Answer from the drawing. Dimensions are ordinates in mm from the lowest x, y and z of the part. Round coordinates to 2 decimals unless told otherwise and drop trailing zeros. Loops run counter-clockwise (first coordinate to the right, second up) from the corner with the lowest first, then second, coordinate; pieces in that order, holes last. Notation, with made-up numbers: M 8,7.5 L 42,7.5 A6 ccw 42,14.5 Z; hole C -5.5,39.25 d4. An arc over 180 degrees is marked long. One line per item, written item: value.
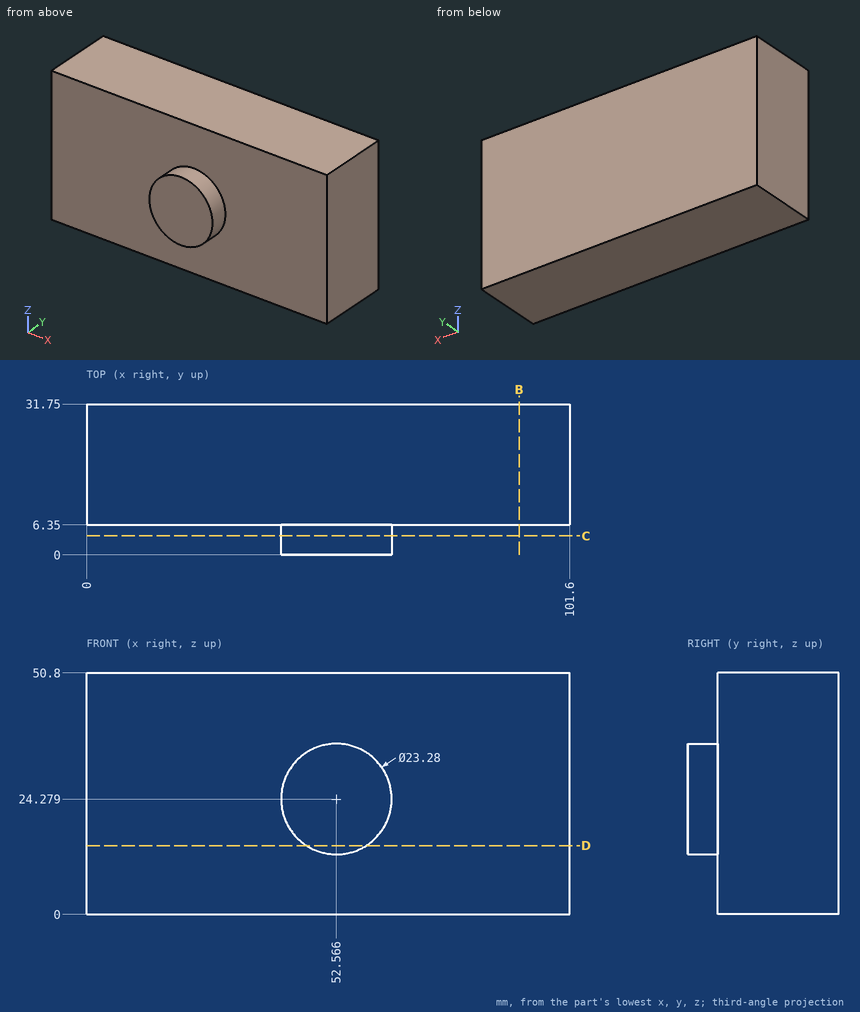
1) Find the intervals of material crossed by probe 1 along Y at (x, z) = (50, 8); probe 2 along X at (y, z) = (3.5, 16) (1 decimal), in increasing order. Write a range as from..to.
Check values:
probe 1: 6.35..31.75
probe 2: 44.4..60.7
2) Find section B-B (x = 91). Give the vertices of the cut face in (y, z).
Check values:
outline: M 6.35,0 L 31.75,0 L 31.75,50.8 L 6.35,50.8 Z
3) Each of these flat-tipped pins is pushed along its axis until it touches: pin 1 (8 mm diameter, centred on x = 81, z = 24.5, fed in from -Y); pin 2 (2 mm diameter, centred on x = 47.5, y = 10.5, fed in from -Z). Where does it stop, or does it pass through?
Check values:
pin 1: y = 6.35
pin 2: z = 0
4) Find section C-C (y = 4). Give the vertices of the cut face in (x, z) (1 decimal).
Check values:
outline: C 52.6,24.3 d23.3
5) Find section D-D (z = 14.5). Give the vertices of the cut face in (x, y), then the cut area to 3 significant figures.
Check values:
outline: M 0,6.35 L 46.25,6.35 L 46.25,0 L 58.88,0 L 58.88,6.35 L 101.6,6.35 L 101.6,31.75 L 0,31.75 Z
area: 2,660 mm2
